```python
from build123d import *

# Parameters (mm, degrees)
F0_W     = 84.257484
F0_H     = 32.520414
F1_DEPTH = 0.5
F5_DEPTH = 2.5
F6_R     = 5.08


with BuildPart() as f1:
    # F0 (on Top) → F1 (new body, symmetric)
    with BuildSketch(Plane.XY):
        Rectangle(F0_W, F0_H)
    extrude(amount=F1_DEPTH, both=True)

    # F2 (on Front) → F3 (revolve)
    with BuildSketch(Plane.XZ):
        with BuildLine():
            Line((0, 0), (-12.19517, 0))
            Line((-12.19517, 0), (-12.19517, -54.693431))
            ThreePointArc((-12.19517, -54.693431), (-18.343741, -76.310214), (0, -89.29472))
            Line((0, -89.29472), (0, 0))
        make_face()
    revolve(axis=Axis((0, 0, -44.64736), (0, 0, -1)))

    # F4 (on Front) → F5 (join, symmetric)
    with BuildSketch(Plane.XZ):
        with BuildLine():
            Line((-30.75086, 508.389294), (-30.75086, 0))
            Line((-30.75086, 0), (30.75086, 0))
            Line((30.75086, 0), (30.75086, 571.142793))
            ThreePointArc((30.75086, 571.142793), (-12.305865, 553.561671), (-30.75086, 510.867883))
            Line((-30.75086, 510.867883), (-30.75086, 508.389294))
        make_face()
        with BuildLine():
            ThreePointArc((-30.75086, 510.867883), (-30.763345, 509.628589), (-30.75086, 508.389294))
            Line((-30.75086, 508.389294), (-30.75086, 510.867883))
        make_face()
    extrude(amount=F5_DEPTH, both=True)

    # F6
    f6_edges = [f1.edges().sort_by_distance(p)[0] for p in [
        (-42.128742, -16.260207, 0),
        (-42.128742, 16.260207, 0),
        (42.128742, 16.260207, 0),
        (42.128742, -16.260207, 0),
    ]]
    fillet(f6_edges, radius=F6_R)


solid = f1.part
```
Could you check a few things on this model? Use its own coordinates, in mm. A direction names the side the tool comes from. Coordinates: 2 decimals unless noted, no trailing zeros. Loops run counter-clockwise (first coordinate to the right, second up) from the corner with the lowest first, then second, coordinate; pieces in that order, holes last.
1) Imagine slicing it at A-A (z = 277.5). List the corners of the cut face in (x, y) for me.
Reported:
outline: (-30.75, -2.5) - (30.75, -2.5) - (30.75, 2.5) - (-30.75, 2.5) - close
2) Which directions (+Z, -Z, +X, -X, +Y, -Y) give clear straight access to the entire face, cutting with the end or side of a thin tool? Please do faces 1 (the face through (9.68, -7.42, -27.98)), 2 (the face through (0, -2.5, 290)), 3 (the face through (0, 2.5, 290)).
Reported:
face 1: none
face 2: +Z, +X, -X, -Y
face 3: +Z, +X, -X, +Y
3) Imagine slicing it at B-B (z = -47). List the corners of the cut face in (x, y) for me, and give its area (3 significant figures).
Reported:
outline: circle Ø24.39 at (0, 0)
area: 467 mm2
4) Will these pins go through, and if not, where does the flat tip stop? pin 1 Ø2.5 at (y, z) = (1, 229.5) entering from +X; pin 2 Ø6 at (y, z) = (2, 350) entering from -X; pin 3 Ø4 at (x, y) = (-13, -4.5) entering from -Z.
Reported:
pin 1: stops at x = 30.75
pin 2: stops at x = -30.75
pin 3: stops at z = -85.34
5) Please list where these lines run through material, in increasing order: line 1 along Z through (x, y) = (18, 12.5); line 2 along Z through (x, y) = (10, -14.5); line 3 along Z through (x, y) = (7, 11.5).
Reported:
line 1: z = -0.5 to 0.5
line 2: z = -78.09 to -61.6, -0.5 to 0.5
line 3: z = -83.88 to -55.81, -0.5 to 0.5
